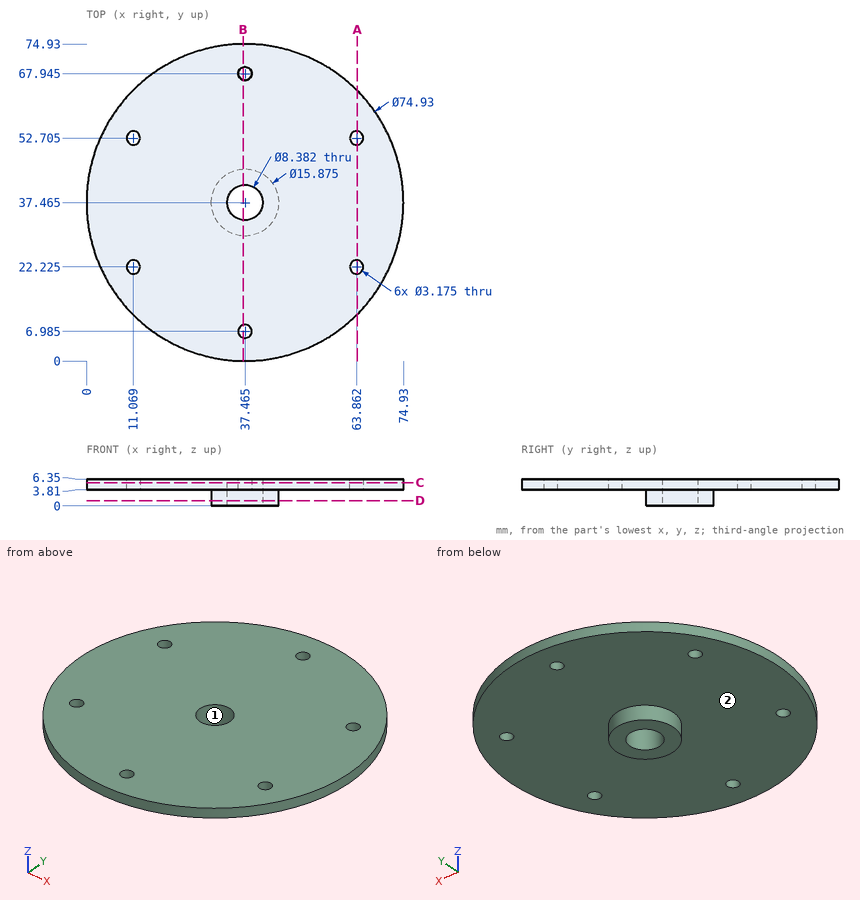
Drawing for the job (mm, zero at the part's lowest x, y, z). Give positions to 0.01 mm unless a question says otherwise; leave off trailing zeros. Write each loop counter-clockwise with the first axis right and the second up, starting at its lowest first coordinate (ties: lowest second). Pieces come first, ordered by that corner, then holes. Notation, with made-up numbers: (2, 47) -> (56, 47) arc R15 cw to (56, 62) -> close; hole circle Ø4 at (4, 77.25). An arc over 180 degrees is marked (long way). Put each result on its own line as item: value. Start each with the question number.
Item 1: Cut at D-D (z = 1.25). List the corners of the cut face in (x, y) (1 decimal).
Item 2: Pin check, flat tips, straight feed: pin 1 Ø12 at (x, y) = (45.5, 62) entering from -Z; pin 2 Ø1.5 at (y, z) = (7.5, 4.5) entering from -X. Stop position of each tip, or through.
Item 3: Wall check: L1, parallel to Z at x = 45.5, y = 53; L2, parallel to X at y = 8, z = 4.25 (1 decimal); L3, parallel to Y at x = 38, z = 2.75 (1 decimal). Give the ranges that are in metal, low to high. Write a range as [from, to].
Item 4: Cut at B-B (x = 37). List the corners of the cut face in (y, z).
Item 5: Cut at A-A (x = 64). List the corners of the cut face in (y, z).
Item 6: Cut at C-C (z = 5.5). State how many separate pieces and enclosed holes the cut face has, then the cut area to 3 significant figures.
Item 7: Pull direction Y, two halves, no side cores. Call the marked faces 1 and 2: pulls with the +Y half, pulls with the -Y half, needs draft (parallel to the pull), parting line crosses it, or undercut.
Answer list:
1. outline: circle Ø15.9 at (37.5, 37.5); hole circle Ø8.4 at (37.5, 37.5)
2. pin 1: stops at z = 3.81
2. pin 2: stops at x = 14.01
3. L1: z = [3.81, 6.35]
3. L2: x = [14.3, 36.2], [38.7, 60.6]
3. L3: y = [29.5, 33.3], [41.6, 45.4]
4. outline: (0, 3.81) -> (5.47, 3.81) -> (5.47, 6.35) -> (0, 6.35) -> close; (8.5, 3.81) -> (29.54, 3.81) -> (29.54, 0) -> (33.3, 0) -> (33.3, 6.35) -> (8.5, 6.35) -> close; (41.63, 0) -> (45.39, 0) -> (45.39, 3.81) -> (66.43, 3.81) -> (66.43, 6.35) -> (41.63, 6.35) -> close; (69.46, 3.81) -> (74.93, 3.81) -> (74.93, 6.35) -> (69.46, 6.35) -> close
5. outline: (11.02, 3.81) -> (20.64, 3.81) -> (20.64, 6.35) -> (11.02, 6.35) -> close; (23.81, 3.81) -> (51.12, 3.81) -> (51.12, 6.35) -> (23.81, 6.35) -> close; (54.29, 3.81) -> (63.91, 3.81) -> (63.91, 6.35) -> (54.29, 6.35) -> close
6. separate pieces: 1
6. enclosed holes: 7
6. area: 4,310 mm2
7. face 1: undercut
7. face 2: needs draft
